Source: CAD feature listing. Evaluate the final solid. Frame: model axes, mm. A direction names the side the tool comes from. Coordinates: 2 decimals unless noted, no trailing zeros. Loops run counter-clockwise (first coordinate to the right, second up) from the corner with the lowest first, then second, coordinate; pieces in that order, holes last.
from build123d import *

# Parameters (mm, degrees)
SKETCH1_R           = 4.25
BOSS_EXTRUDE1_DEPTH = 5.25
CUT_EXTRUDE1_DEPTH  = 3.6
SKETCH3_R           = 2
BOSS_EXTRUDE2_DEPTH = 10


with BuildPart() as part:
    # Sketch1 → Boss-Extrude1 (new body)
    with BuildSketch(Plane(origin=(0, 0, 0), x_dir=(0, 0, -1), z_dir=(1, 0, 0))):
        Circle(SKETCH1_R)
    extrude(amount=BOSS_EXTRUDE1_DEPTH)

    # Sketch2 → Cut-Extrude1 (cut)
    with BuildSketch(Plane(origin=(5.25, 0, 0), x_dir=(0, 0, -1), z_dir=(1, 0, 0))):
        Polygon((0, 2.309401077), (-2, 1.154700538), (-2, -1.154700538), (0, -2.309401077), (2, -1.154700538), (2, 1.154700538), align=None)
    extrude(amount=-CUT_EXTRUDE1_DEPTH, mode=Mode.SUBTRACT)

    # Sketch3 → Boss-Extrude2 (add)
    with BuildSketch(Plane.ZY):
        Circle(SKETCH3_R)
    extrude(amount=BOSS_EXTRUDE2_DEPTH)


solid = part.part
Q1. Line query: line 1 along X through (y, z) = (3.25, 2); line 2 along X through (y, z) = (-1.5, -0.25); line 3 along Y through (x, z) = (2.5, 3.75). Output: solid intervals per line, ascending.
Q2. Section D-D, the plane z = -1.75. Return the cut outline in (x, y), plus the area to 3 significant figures.
Q3. Section B-B, the plane y = 0. Return the cut outline in (x, z), plus the area to 3 significant figures.
Q4. Section C-C, the plane x = -2.75. Return the cut outline in (y, z).
Q5. Section A-A, the plane x = 4. Return the cut outline in (y, z).
Q6. Draft query along Y for faces 4 (the flat face through (-10, 0, 0)), 5 (the flat face through (1.65, 0, 0)), 6 (the cylindrical face through (-5, -2, 0)). Return one class per face: +Y half, -Y half, draft (parallel to the pull), parting line (faces both ways), or undercut.
Q7. Access query for faces 1 (the cylindrical face through (2.588, 3.584, -2.285)), 2 (the flat face through (3, 0, 2)), 3 (the flat face through (0, -1, -2)). Directions: +Z, -Z, +X, -X, +Y, -Y. A direction counts if a zero-diameter tool reaches every point of the face in a straight line with its end or side. Return the directions, or none.
Q8. Contact query for flat-ended pins moving along their axis: pin 1 Ø3 at (y, z) = (1, 0.5) entering from +X; pin 2 Ø1 at (x, z) = (-2, -1) entering from -Y; pin 3 Ø5 at (y, z) = (-3, 3.5) entering from -X. Output: stop coordinate, or through.
Derived:
1. line 1: x = 0 to 5.25
1. line 2: x = -10 to 1.65
1. line 3: y = -2 to 2
2. outline: (-10, -0.97) - (0, -0.97) - (0, -3.87) - (5.25, -3.87) - (5.25, -1.3) - (1.65, -1.3) - (1.65, 1.3) - (5.25, 1.3) - (5.25, 3.87) - (0, 3.87) - (0, 0.97) - (-10, 0.97) - close
2. area: 50.7 mm2
3. outline: (-10, -2) - (0, -2) - (0, -4.25) - (5.25, -4.25) - (5.25, -2) - (1.65, -2) - (1.65, 2) - (5.25, 2) - (5.25, 4.25) - (0, 4.25) - (0, 2) - (-10, 2) - close
3. area: 70.2 mm2
4. outline: circle Ø4 at (0, 0)
5. outline: circle Ø8.5 at (0, 0); hole (-2.31, 0) - (-1.15, -2) - (1.15, -2) - (2.31, 0) - (1.15, 2) - (-1.15, 2) - close
6. face 4: draft
6. face 5: undercut
6. face 6: parting line
7. face 1: +X, -X
7. face 2: +X
7. face 3: -X
8. pin 1: stops at x = 5.25
8. pin 2: stops at y = -1.94
8. pin 3: stops at x = 0
